The listing builds one solid part. Answer for the finished solid, in the listing's coordinates (mm). A direction names the side the tool comes from. Coordinates: 2 decimals unless noted, no trailing zeros. Loops run counter-clockwise (first coordinate to the right, second up) from the corner with the lowest first, then second, coordinate; pieces in that order, holes last. Notation, with made-up numbers: (1, 62) -> (19, 62) arc R14 cw to (19, 73) -> close; hole circle Ø11 at (7.5, 15). An arc over 180 degrees is marked (long way). Answer in a Markdown table with one row per item.
```python
from build123d import *

# Parameters (mm, degrees)
F0_W     = 52.5193866342
F0_H     = 111.6036958992
F1_DEPTH = 50.8
F2_T     = -6.35
F3_DEPTH = 12.7


with BuildPart() as f1:
    # F0 (on Top) → F1 (new body)
    with BuildSketch(Plane.XY):
        with Locations((1.9489629194, 0.4103090614)):
            Rectangle(F0_W, F0_H)
    extrude(amount=F1_DEPTH)

    # F2
    f2_openings = [f1.faces().sort_by_distance(p)[0] for p in [
        (1.948963, -55.391539, 25.4),
    ]]
    offset(amount=F2_T, openings=f2_openings)

    # F3 (add): faces of the model
    f3_faces = [f1.faces().sort_by_distance(p)[0] for p in [
        (1.9489629194, 56.212157011, 25.4),
        (1.9489629194, 49.862157011, 25.4),
    ]]
    extrude(f3_faces, amount=-F3_DEPTH, dir=(0, 1, 0))


solid = f1.part
```
Item 1: A tool of negligible diameter and unlimited length cuts with its end or side. For faces 1 (the face through (-17.961, -10, 25)), 2 (the face through (28.209, 1, 25)), from which of +Z, -Z, +X, -X, +Y, -Y can it reach the whole face along a straight path? Write none if from no direction.
Findings below:
| item | result |
|---|---|
| face 1 | -Y |
| face 2 | +Z, -Z, +X, +Y, -Y |
Item 2: Determine the mould class of faces 3 (the face through (2, 1, 0)), 4 (the face through (2, -8, 6.35)), 5 (the face through (-24.311, 1, 25)), 6 (the face through (21.859, -10, 25)) for opening direction X: +X half, -X half, draft (parallel to the pull), parting line (faces both ways), or undercut.
Findings below:
| item | result |
|---|---|
| face 3 | draft |
| face 4 | undercut |
| face 5 | -X half |
| face 6 | undercut |
Item 3: A cutting plane is placed at A-A, the plane x = 17. Determine the outline of the cut face in (y, z).
Findings below:
| item | result |
|---|---|
| outline | (-55.39, 0) -> (56.21, 0) -> (56.21, 50.8) -> (-55.39, 50.8) -> (-55.39, 44.45) -> (37.16, 44.45) -> (37.16, 6.35) -> (-55.39, 6.35) -> close |
Item 4: A cutting plane is placed at B-B, the plane z = 38. Determine the outline of the cut face in (x, y), plus the area to 3 significant figures.
Findings below:
| item | result |
|---|---|
| outline | (-24.31, -55.39) -> (-17.96, -55.39) -> (-17.96, 37.16) -> (21.86, 37.16) -> (21.86, -55.39) -> (28.21, -55.39) -> (28.21, 56.21) -> (-24.31, 56.21) -> close |
| area | 2,180 mm2 |
Item 5: Find the intervals of material crossed by probe 1 along X at (y, z) = (24.5, 6.5); probe 2 along Z at (x, y) = (18, -15.5); probe 3 along Y at (x, z) = (-9, 10.5), in increasing order.
Findings below:
| item | result |
|---|---|
| probe 1 | x = -24.31 to -17.96, 21.86 to 28.21 |
| probe 2 | z = 0 to 6.35, 44.45 to 50.8 |
| probe 3 | y = 37.16 to 56.21 |
Item 6: A cutting plane is placed at C-C, the plane y = -15.5. Determine the outline of the cut face in (x, z).
Findings below:
| item | result |
|---|---|
| outline | (-24.31, 0) -> (28.21, 0) -> (28.21, 50.8) -> (-24.31, 50.8) -> close; hole (-17.96, 6.35) -> (21.86, 6.35) -> (21.86, 44.45) -> (-17.96, 44.45) -> close |
Item 7: A flat-ended cylindrical pin translates along its axis: pin 1 Ø11.5 at (x, z) = (4.5, 17.5) entering from -Y. Find the tip coordinate at first contact, or state that the pin passes through.
Findings below:
| item | result |
|---|---|
| pin 1 | stops at y = 37.16 |
